Here's the drawing with two shaded views (mm, measured from the low corner). I have some questions. Coordinates: 2 decimals unless noted, no trailing zeros. Write each loop counter-clockwise with the first axis right and the second up, starting at its lowest first coordinate (ties: lowest second). Pieces come first, ordered by that corner, then holes. Notation, with made-up numbers: (24.25, 61) - (52.25, 61) arc R16 ccw to (52.25, 92) - close; hole circle Ø1 at (26, 10). An arc over 180 degrees is marked (long way). Answer in a Markdown table with one row per item. Add a question column.
Item 1: Imagine slicing it at B-B (y = 67.6). Please give me the cut outline in (x, z), plus the area to 3 significant figures.
Item 2: Imagine slicing it at D-D (y = 51.5). Please give me the cut outline in (x, z), plus the area to 3 significant figures.
Item 3: Imagine slicing it at A-A (z = 3.1). Please give me the cut outline in (x, y), plus the area to 3 significant figures.
Item 4: I'm going to push flat-ended pins straight in: pin 1 (1.6 mm diameter, centred on x = 32, z = 1.5, fed in from +Y); pin 2 (3 mm diameter, centred on x = 90.35, y = 2.6, fed in from -Z); pin 3 (3 mm diameter, centred on x = 41, y = 29, fed in from +Z). Where does each tip first touch, or does it pass through?
Item 5: We'd pull the mould along Y, two halves only. Please class the marked faces 1 and 2: +Y half, -Y half, draft (parallel to the pull), parting line (faces both ways), or undercut.
Item 6: Imagine slicing it at C-C (x = 90.35). Please give me the cut outline in (y, z).
Item 7: If I drill on probe 1 along Y at (x, z) = (2.4, 2.6); probe 2 along Y at (x, z) = (2.4, 1.05); probe 3 along X at (y, z) = (13, 4.75), over which ranges is the centre line in solid material (lowest first)? Write a range as from..to.
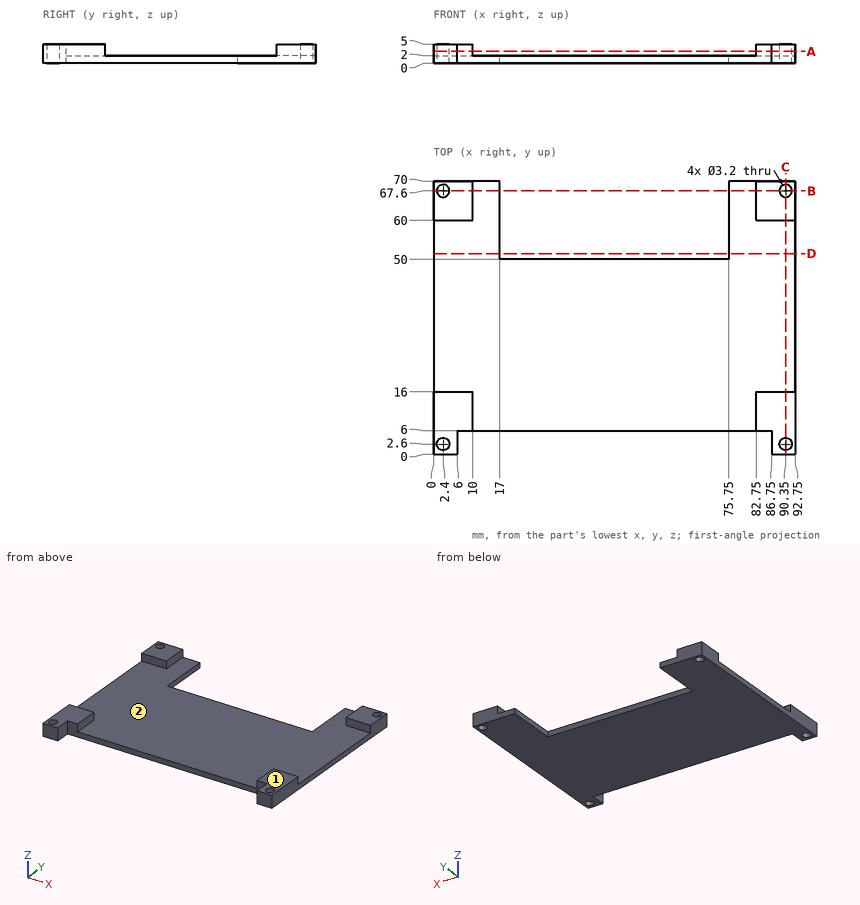
Here are the results:
| question | item | result |
|---|---|---|
| 1 | outline | (0, 0) - (0.8, 0) - (0.8, 5) - (0, 5) - close; (4, 0) - (17, 0) - (17, 2) - (10, 2) - (10, 5) - (4, 5) - close; (75.75, 0) - (88.75, 0) - (88.75, 5) - (82.75, 5) - (82.75, 2) - (75.75, 2) - close; (91.95, 0) - (92.75, 0) - (92.75, 5) - (91.95, 5) - close |
| 1 | area | 96.0 mm2 |
| 2 | outline | (0, 0) - (17, 0) - (17, 2) - (0, 2) - close; (75.75, 0) - (92.75, 0) - (92.75, 2) - (75.75, 2) - close |
| 2 | area | 68.0 mm2 |
| 3 | outline | (0, 0) - (6, 0) - (6, 6) - (10, 6) - (10, 16) - (0, 16) - close; (0, 60) - (10, 60) - (10, 70) - (0, 70) - close; (82.75, 6) - (86.75, 6) - (86.75, 0) - (92.75, 0) - (92.75, 16) - (82.75, 16) - close; (82.75, 60) - (92.75, 60) - (92.75, 70) - (82.75, 70) - close; hole circle Ø3.2 at (2.4, 2.6); hole circle Ø3.2 at (2.4, 67.6); hole circle Ø3.2 at (90.35, 2.6); hole circle Ø3.2 at (90.35, 67.6) |
| 3 | area | 440 mm2 |
| 4 | pin 1 | stops at y = 50 |
| 4 | pin 2 | passes through |
| 4 | pin 3 | stops at z = 2 |
| 5 | face 1 | draft |
| 5 | face 2 | undercut |
| 6 | outline | (0, 0) - (1, 0) - (1, 5) - (0, 5) - close; (4.2, 0) - (66, 0) - (66, 5) - (60, 5) - (60, 2) - (16, 2) - (16, 5) - (4.2, 5) - close; (69.2, 0) - (70, 0) - (70, 5) - (69.2, 5) - close |
| 7 | probe 1 | y = 0..1, 4.2..16, 60..66, 69.2..70 |
| 7 | probe 2 | y = 0..1, 4.2..66, 69.2..70 |
| 7 | probe 3 | x = 0..10, 82.75..92.75 |
